Design review of the part built by this model. Coordinates are the model's own, in mm. A direction names the side the tool comes from. Round coordinates to 2 decimals unless told otherwise and drop trailing zeros. Order: outer loops, then holes, each group sorted by start corner. A loop starts at its lowest first (then second) coordinate and runs counter-clockwise, first axis right, second up. Notation, with made-up numbers: (-13.5, 45.5) - (44.5, 45.5) arc R11 cw to (44.5, 58.5) - close; hole circle Ø9 at (85, 55.5). An arc over 180 degrees is marked (long way). Write item = value, one per line.
from build123d import *

# Parameters (mm, degrees)
SKETCH3_R               = 4
BOSS_EXTRUDE1_DEPTH     = 25
BOSS_EXTRUDE2_START     = 25
SKETCH3_5_R             = 3
BOSS_EXTRUDE2_DEPTH     = 8
FILLET1_R               = 1
CUT_EXTRUDE1_DEPTH      = 17
CUT_EXTRUDE1_DEPTH_BACK = 46.978255774
SKETCH15_R              = 1.8
FILLET3_R               = 1


with BuildPart() as part:
    # Sketch1 → Revolve1 (revolve)
    with BuildSketch(Plane.XY, mode=Mode.PRIVATE) as revolve1_sk:
        Polygon((0, 20), (0, 0), (25, 0), (25, 5), (10, 5), (10, 20), align=None)
    revolve(revolve1_sk.sketch.rotate(Axis((0, 20, 0), (0, -1, 0)), 90), axis=Axis((0, 20, 0), (0, -1, 0)))

    # Sketch3 → Boss-Extrude1 (add)
    with BuildSketch(Plane(origin=(0, 0, 0), x_dir=(0, 0, -1), z_dir=(1, 0, 0))):
        with Locations(Location((0, 12, 0), (0, 0, 180))):
            Circle(SKETCH3_R)
    extrude(amount=BOSS_EXTRUDE1_DEPTH)

    # Sketch3<5> → Boss-Extrude2 (add)
    with BuildSketch(Plane(origin=(0, 0, 0), x_dir=(0, 0, -1), z_dir=(1, 0, 0)).offset(BOSS_EXTRUDE2_START)):
        with Locations((0, 12)):
            Circle(SKETCH3_5_R)
    extrude(amount=BOSS_EXTRUDE2_DEPTH)

    # Fillet1
    fillet1_edges = [part.edges().sort_by_distance(p)[0] for p in [
        (0, 5, -25),
        (0, 0, -25),
    ]]
    fillet(fillet1_edges, radius=FILLET1_R)

    # Sketch11 → Cut-Revolve10 (revolve, cut)
    with BuildSketch(Plane.XY, mode=Mode.PRIVATE) as cut_revolve10_sk:
        with BuildLine():
            Line((0, 4), (0, 0))
            Line((0, 0), (22.072872435, 0))
            ThreePointArc((22.072872435, 0), (11.216213299, 2.992049146), (0, 4))
        make_face()
    revolve(cut_revolve10_sk.sketch.rotate(Axis((0, 0, 0), (0, 1, 0)), 90), axis=Axis((0, 0, 0), (0, 1, 0)), mode=Mode.SUBTRACT)

    # Sketch15 → Cut-Extrude1 (cut, two sides: drawn at the far end of the back side and taken through both)
    with BuildSketch(Plane(origin=(0, 0, 0), x_dir=(1, 0, 0), z_dir=(0, 1, 0)).offset(-CUT_EXTRUDE1_DEPTH_BACK)):
        with Locations(Location((0, 0, 0), (0, 0, 270))):
            Circle(SKETCH15_R)
    extrude(amount=CUT_EXTRUDE1_DEPTH + CUT_EXTRUDE1_DEPTH_BACK, mode=Mode.SUBTRACT)

    # Sketch16 → Cut-Revolve12 (revolve, cut)
    with BuildSketch(Plane.XY, mode=Mode.PRIVATE) as cut_revolve12_sk:
        Polygon((33, 15), (33, 13.5), (15.503373698, 16), (33, 16), align=None)
    revolve(cut_revolve12_sk.sketch.rotate(Axis((33, 12, 0), (-1, 0, 0)), 270), axis=Axis((33, 12, 0), (-1, 0, 0)), mode=Mode.SUBTRACT)

    # Sketch17 → Cut-Revolve13 (revolve, cut)
    with BuildSketch(Plane.XY, mode=Mode.PRIVATE) as cut_revolve13_sk:
        Polygon((33, 12.6), (33, 12), (0, 12), (0, 14.8), (15.503373698, 14.8), (30.900404844, 12.6), align=None)
    revolve(cut_revolve13_sk.sketch.rotate(Axis((33, 12, 0), (-1, 0, 0)), 90), axis=Axis((33, 12, 0), (-1, 0, 0)), mode=Mode.SUBTRACT)

    # Fillet3
    fillet3_edges = [part.edges().sort_by_distance(p)[0] for p in [
        (9.16515139, 12, -4),
        (15.503373698, 12, -4),
        (33, 12, -1.5),
        (0, 5, -10),
    ]]
    fillet(fillet3_edges, radius=FILLET3_R)


solid = part.part
Item 1: For line 1 along Z through (x, y) = (9.75, 12); line 2 along Z through (x, y) = (32.05, 12); line 3 along Y through (x, z) = (12.5, 0), list the stretches that pass through material, from the lowest coordinate up. Write a range as [from, to].
Data:
line_1 = [-4, -2.8], [2.8, 4]
line_2 = [-1.64, -0.6], [0.6, 1.64]
line_3 = [2.75, 5], [8, 9.2], [14.8, 16]
Item 2: Insertion check: P1, Ø6, axis at x = 15, z = 10.5, coming from the -Y side; P2, Ø6, axis at y = 10.5, z = -7.5, coming from the -X side; P3, Ø5, axis at x = 26.5, y = 15.5, coming from the +Z side; P4, Ø8, axis at x = 11, z = -4, coming from the +Y side. Each pin has a flat end and moves straight along its axis. Give the tip position at first contact, or say it passes through.
Data:
P1 = 0.28
P2 = -8.93
P3 = 2.28
P4 = 20
Item 3: Take a section at B-B, the plane x = 29.5. State the section outline as (y, z) points, and give its area (3 significant figures).
Data:
outline = circle Ø4 at (12, 0); hole circle Ø1.6 at (12, 0)
area = 10.6 mm2
Item 4: The part is to be moulded in two halves that separate along Y. For faces 1 (the face through (-7.509, 2.521, 23.846)), 2 (the face through (12.575, 8.627, 2.15)), 3 (the face through (31.965, 12.586, 0.13)), 4 (the face through (0, 20, 0)), say which applies: +Y half, -Y half, draft (parallel to the pull), parting line (faces both ways), or undercut.
Data:
face_1 = draft
face_2 = undercut
face_3 = undercut
face_4 = +Y half
Item 5: Take a section at A-A, the plane x = 12.5. Count the separate pieces of the cut face and the enclosed holes in it, and give its area (3 significant figures).
Data:
separate_pieces = 2
enclosed_holes = 1
area = 174 mm2
Item 6: For faces 5 (the face through (23.31, 10.33, 0.22)), 6 (the face through (7, 0, -21.2)), 7 (the face through (0, 17, 0)), list the 3-axis set-ups (+Z, -Z, +X, -X, +Y, -Y) from which the entire face can be reached by the end or side of a thin tool; tool diameter is ignored.
Data:
face_5 = none
face_6 = +Z, -Z, +X, -X, -Y
face_7 = -Y
